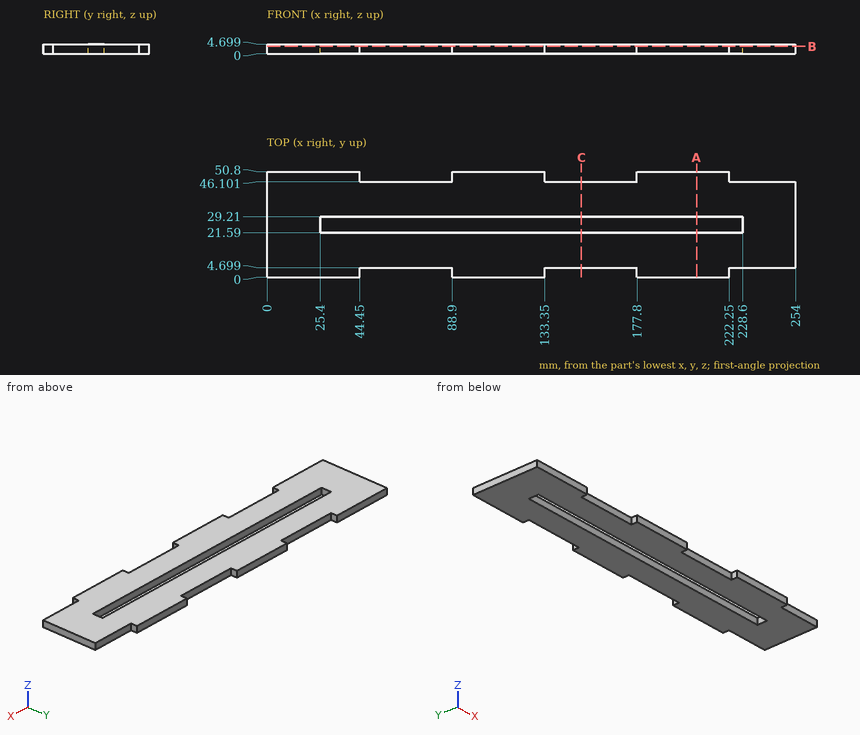
Input: dimensioned drawing with shaded views. Units: mm. Origin: part minimum x, y, z. Give positions to 0.01 mm unless a question says otherwise; leave off trailing zeros. Order: outer loops, then holes, each group sorted by start corner. A loop starts at its lowest first (then second) coordinate and runs counter-clockwise, first axis right, second up. Notation, with made-up numbers: (67.5, -15) -> (100.5, -15) arc R31 cw to (100.5, 19) -> close; hole circle Ø1 at (62, 18.25). An arc over 180 degrees is marked (long way). Use one line per item in the form item = value.
1) First-contact query: pin 1 Ø2.5 at (x, z) = (233.5, 3) entering from -Y; pin 2 Ø1.4 at (x, z) = (93, 3) entering from -Y; pin 3 Ø1.4 at (x, z) = (85.5, 1.5) entering from +Y. Flat tips, straight axial feed; report the tip coordinate or a pass-through.
Response values:
pin_1 = 4.7
pin_2 = 0
pin_3 = 46.1
2) Line query: probe 1 along X at (y, z) = (48, 2.2); probe 2 along Y at (x, z) = (133, 0.3); probe 3 along Y at (x, z) = (138.5, 2.25). Output: solid intervals per line, ascending.
Response values:
probe_1 = 0 to 44.45, 88.9 to 133.35, 177.8 to 222.25
probe_2 = 0 to 21.59, 29.21 to 50.8
probe_3 = 4.7 to 21.59, 29.21 to 46.1
3) Section A-A, the plane x = 206.5. Return loops of the section in (y, z), and give its area (3 significant figures).
Response values:
outline = (0, 0) -> (21.59, 0) -> (21.59, 4.7) -> (0, 4.7) -> close; (29.21, 0) -> (50.8, 0) -> (50.8, 4.7) -> (29.21, 4.7) -> close
area = 203 mm^2
4) Section C-C, the plane x = 151. Return loops of the section in (y, z).
Response values:
outline = (4.7, 0) -> (21.59, 0) -> (21.59, 4.7) -> (4.7, 4.7) -> close; (29.21, 0) -> (46.1, 0) -> (46.1, 4.7) -> (29.21, 4.7) -> close
5) Section B-B, the plane z = 3.55. Return loops of the section in (x, y), and give its area (3 significant figures).
Response values:
outline = (0, 0) -> (44.45, 0) -> (44.45, 4.7) -> (88.9, 4.7) -> (88.9, 0) -> (133.35, 0) -> (133.35, 4.7) -> (177.8, 4.7) -> (177.8, 0) -> (222.25, 0) -> (222.25, 4.7) -> (254, 4.7) -> (254, 46.1) -> (222.25, 46.1) -> (222.25, 50.8) -> (177.8, 50.8) -> (177.8, 46.1) -> (133.35, 46.1) -> (133.35, 50.8) -> (88.9, 50.8) -> (88.9, 46.1) -> (44.45, 46.1) -> (44.45, 50.8) -> (0, 50.8) -> close; hole (25.4, 21.59) -> (228.6, 21.59) -> (228.6, 29.21) -> (25.4, 29.21) -> close
area = 10,200 mm^2
